Design review of the part built by this model. Coordinates are the model's own, in mm. Give positions to 0.01 mm unless a question says otherwise; leave off trailing zeros. Order: outer loops, then holes, each group sorted by start corner. A loop starts at its lowest first (then second) coordinate and runs counter-clockwise, first axis right, second up. Notation, with made-up numbers: (-14.75, -34) -> (-3.75, -34) arc R34 ccw to (-3.75, 0) -> close; hole circle Ø11 at (86.25, -29.75). An arc over 180 degrees is marked (long way). One line per item, written item: value. Start each with the question number.
1) Consider section B-B (x = 50.8). State the section outline as (y, z) points.
2) Consider section D-D (x = -9.5). State the section outline as (y, z) points, plus the area to 3 significant figures.
3) Consider section C-C (y = 37). State the section outline as (x, z) points, plus the area to 3 significant figures.
4) Wall thickness on line 1 along Y through (x, z) = (50.8, 5.5); line 2 along Y through (x, z) = (50.8, 3.5); line 3 along Y through (x, z) = (-29.5, 6.25): over which ranges is each line inside the solid? List them lowest first. Write a range as from..to.
5) The part is to be moulded in two halves that separate along X. For faces 1 (the face through (57.43, -57.47, 3.55)), 2 (the face through (-1, -58.181, 3)), 3 (the face through (52.08, -48.79, 3.55)), say which applies: released by +X, released by -X, zero draft, split by the parting line, or undercut.
6) Consider section A-A (y = -50.8). State the section outline as (x, z) points, plus the area to 3 significant figures.
7) For pin 1 (8 mm diameter, centred on x = 11.5, y = 37, fed in from +Z); pin 2 (6 mm diameter, centred on x = 50.8, y = -50.8, fed in from +Z); pin 3 (3 mm diameter, centred on x = 50.8, y = 50.8, fed in from -Z), all flat-tipped, find the tip position at first contact; note any pin that passes through.
Autodesk Fusion 360 part; units mm, degrees
ref_plane "WorkPlane1" through (0, 0, 7) normal (0, 0, 1) x (1, 0, 0)
sketch "Base Plate Sketch" plane through (0, 0, 0) normal (0, 0, 1) x (1, 0, 0)
  line L0 (-58.1813, -58.1813) -> (58.1813, -58.1813)
  line L1 (58.1813, -58.1813) -> (58.1813, 59)
  line L2 (58.1813, 59) -> (-58.1813, 59)
  line L3 (-58.1813, 59) -> (-58.1813, -58.1813)
extrude "Base Plate" add sketch "Base Plate Sketch" along normal blind 7
fillet "Fillet1" radius 2.5 4 edges at (-58.1813, 59, 3.5) (58.1813, 59, 3.5) (58.1813, -58.1813, 3.5) (-58.1813, -58.1813, 3.5)
sketch "Wafer Nest Pocket Sketch" plane through (0, 0, 7) normal (0, 0, 1) x (1, 0, 0)
  line L0 (-52.5, -47.4607) -> (52.5, -47.4607)
  line L1 (52.5, -47.4607) -> (52.5, 54)
  line L2 (52.5, 54) -> (-52.5, 54)
  line L3 (-52.5, 54) -> (-52.5, -47.4607)
extrude "Wafer Nest Pocket" cut sketch "Wafer Nest Pocket Sketch" against normal blind 2
sketch "Front-Center Access Relief Sketch" plane through (0, 0, 7) normal (0, 0, 1) x (1, 0, 0)
  line L0 (-7.5, -59.1812) -> (7.5, -59.1812)
  line L1 (7.5, -59.1812) -> (7.5, -44.4607)
  line L2 (7.5, -44.4607) -> (-7.5, -44.4607)
  line L3 (-7.5, -44.4607) -> (-7.5, -59.1812)
extrude "Front-Center Access Relief" cut sketch "Front-Center Access Relief Sketch" against normal blind 2
sketch "Rear-Center Access Relief Sketch" plane through (0, 0, 7) normal (0, 0, 1) x (1, 0, 0)
  line L0 (-7.5, 51) -> (7.5, 51)
  line L1 (7.5, 51) -> (7.5, 60)
  line L2 (7.5, 60) -> (-7.5, 60)
  line L3 (-7.5, 60) -> (-7.5, 51)
extrude "Rear-Center Access Relief" cut sketch "Rear-Center Access Relief Sketch" against normal blind 2
sketch "X Datum Square Sketch (165 deg / 9:30)" plane through (0, 0, 7) normal (0, 0, 1) x (1, 0, 0)
  line L0 (-56.2622, 20.1998) -> (-48.2622, 20.1998)
  line L1 (-48.2622, 20.1998) -> (-48.2622, 13.1998)
  arc A0 (-49.2622, 12.1998) -> (-48.2622, 13.1998) centre (-49.2622, 13.1998) ccw
  line L2 (-49.2622, 12.1998) -> (-56.2622, 12.1998)
  line L3 (-56.2622, 12.1998) -> (-56.2622, 20.1998)
extrude "X Datum Square (165 deg / 9:30, rounded corner)" add sketch "X Datum Square Sketch (165 deg / 9:30)" against normal blind 2
sketch "Left Wall Flush Above X-Datum Sketch" plane through (0, 0, 7) normal (0, 0, 1) x (1, 0, 0)
  line L0 (-52.5, 20.1998) -> (-48.2622, 20.1998)
  line L1 (-48.2622, 20.1998) -> (-48.2622, 54)
  line L2 (-48.2622, 54) -> (-52.5, 54)
  line L3 (-52.5, 54) -> (-52.5, 20.1998)
extrude "Left Wall Flush Above X-Datum" add sketch "Left Wall Flush Above X-Datum Sketch" against normal blind 2
sketch "Corner Clip (dowel -50.8, +50.8) Sketch" plane through (0, 0, 7) normal (0, 0, 1) x (1, 0, 0)
  line L0 (-52.5, 44.9187) -> (-44.9187, 44.9187)
  line L1 (-44.9187, 44.9187) -> (-44.9187, 54)
  line L2 (-44.9187, 54) -> (-52.5, 54)
  line L3 (-52.5, 54) -> (-52.5, 44.9187)
extrude "Corner Clip (dowel -50.8, +50.8)" add sketch "Corner Clip (dowel -50.8, +50.8) Sketch" against normal blind 2
sketch "Corner Clip (dowel +50.8, +50.8) Sketch" plane through (0, 0, 7) normal (0, 0, 1) x (1, 0, 0)
  line L0 (44.9187, 44.9187) -> (52.5, 44.9187)
  line L1 (52.5, 44.9187) -> (52.5, 54)
  line L2 (52.5, 54) -> (44.9187, 54)
  line L3 (44.9187, 54) -> (44.9187, 44.9187)
extrude "Corner Clip (dowel +50.8, +50.8)" add sketch "Corner Clip (dowel +50.8, +50.8) Sketch" against normal blind 2
sketch "Outer Front Left Dowel Bore Sketch" plane through (0, 0, 7) normal (0, 0, 1) x (1, 0, 0)
  circle A0 centre (-50.8, -50.8) radius 2.3813
extrude "Outer Front Left Dowel Bore" cut sketch "Outer Front Left Dowel Bore Sketch" against normal blind 7
sketch "Outer Front Right Dowel Bore Sketch" plane through (0, 0, 7) normal (0, 0, 1) x (1, 0, 0)
  circle A0 centre (50.8, -50.8) radius 2.3813
extrude "Outer Front Right Dowel Bore" cut sketch "Outer Front Right Dowel Bore Sketch" against normal blind 7
sketch "Outer Rear Left Dowel Bore Sketch" plane through (0, 0, 7) normal (0, 0, 1) x (1, 0, 0)
  circle A0 centre (-50.8, 50.8) radius 2.3813
extrude "Outer Rear Left Dowel Bore" cut sketch "Outer Rear Left Dowel Bore Sketch" against normal blind 7
sketch "Outer Rear Right Dowel Bore Sketch" plane through (0, 0, 7) normal (0, 0, 1) x (1, 0, 0)
  circle A0 centre (50.8, 50.8) radius 2.3813
extrude "Outer Rear Right Dowel Bore" cut sketch "Outer Rear Right Dowel Bore Sketch" against normal blind 7
equation "gridPitch = 25.4 mm"
equation "indexMove = 50.8 mm"
equation "outerPinPatternSpan = 101.6 mm"
equation "dowelDiameter = 4.7625 mm"
equation "dowelHoleDiameter = 4.7625 mm"
equation "plateEdgeMargin = 5.0 mm"
equation "plateWidth = 116.3625 mm"
equation "plateHeight = 117.18125 mm"
equation "baseThickness = 7.0 mm"
equation "pocketDepth = 2.0 mm"
equation "nestClearanceSide = 2.5 mm"
equation "nestClearanceRear = 4.0 mm"
equation "filletRadius = 2.5 mm"
equation "primaryFlatClearance = 0.175 mm"
equation "xDatumSize = 8.0 mm"
equation "nestReliefWidth = 15.0 mm"
equation "nestOffsetX = 0.0 mm"
equation "nestOffsetY = 0.0 mm"
Checked values:
1. outline: (-58.18, 0) -> (-53.18, 0) -> (-53.18, 7) -> (-58.18, 7) -> close; (-48.42, 0) -> (48.42, 0) -> (48.42, 7) -> (44.92, 7) -> (44.92, 5) -> (-47.46, 5) -> (-47.46, 7) -> (-48.42, 7) -> close; (53.18, 0) -> (59, 0) -> (59, 7) -> (53.18, 7) -> close
2. outline: (-58.18, 0) -> (59, 0) -> (59, 7) -> (54, 7) -> (54, 5) -> (-47.46, 5) -> (-47.46, 7) -> (-58.18, 7) -> close
2. area: 617 mm^2
3. outline: (-58.18, 0) -> (58.18, 0) -> (58.18, 7) -> (52.5, 7) -> (52.5, 5) -> (-48.26, 5) -> (-48.26, 7) -> (-58.18, 7) -> close
3. area: 613 mm^2
4. line 1: y = -58.18..-53.18, -48.42..-47.46, 44.92..48.42, 53.18..59
4. line 2: y = -58.18..-53.18, -48.42..48.42, 53.18..59
4. line 3: y = -58.18..-47.46, 54..59
5. face 1: released by +X
5. face 2: zero draft
5. face 3: undercut
6. outline: (-58.18, 0) -> (-53.18, 0) -> (-53.18, 7) -> (-58.18, 7) -> close; (-48.42, 0) -> (48.42, 0) -> (48.42, 7) -> (7.5, 7) -> (7.5, 5) -> (-7.5, 5) -> (-7.5, 7) -> (-48.42, 7) -> close; (53.18, 0) -> (58.18, 0) -> (58.18, 7) -> (53.18, 7) -> close
6. area: 718 mm^2
7. pin 1: stops at z = 5
7. pin 2: stops at z = 7
7. pin 3: passes through
